Study the drawing (mm; zero at the part's minimum x, y, z) and answer. A direction names the side the tool comes from. Round coordinates to 2 decimals unless told otherwise and drop trailing zeros. Write each loop counter-clockwise with the first axis right and the second up, starting at its lowest first coordinate (ties: lowest second). Pieces come first, ordered by that corner, then holes. Notation, with made-up numbers: (-17, -35.75) - (-13, -35.75) arc R23 ccw to (-13, -6.75) - close; hole circle Ø10 at (53, 8). An arc over 180 degrees is marked (long way). Use one line per item in the form item = value. Start each with the question number.
1) The part is cut by section B-B, the plane y = 18. Give the vertices of the cut face in (x, z), plus the area to 3 significant figures.
2) This flat-tipped pin is pushed along its axis until it touches: pin 1 (11 mm diameter, centred on x = 30, z = 7.5, fed in from +Y). Where does it stop, or does it pass through?
3) The part is cut by section D-D, the plane x = 112.5. Give the vertices of the cut face in (y, z).
4) Consider line 1 along X through (y, z) = (85.5, 46); line 2 along X through (y, z) = (32.5, 38); line 3 along X through (y, z) = (59, 7.5). Determine where each line is inside the solid, lowest interval first. Write a range as from..to.
5) The part is cut by section A-A, the plane x = 43. Give the vertices of the cut face in (y, z), plus the area to 3 significant figures.
6) For the marked faces 4, 5 and 6, determine the directions among +Z, -Z, +X, -X, +Y, -Y from which every point of the face is accessible in a straight line to the end or side of a thin tool.
7) The part is cut by section C-C, the plane z = 35. Give the vertices of the cut face in (x, y).
8) For a pull along Z with two mould halves and no side action, classify the marked faces 1, 2 and 3 as released by +Z, released by -Z, zero draft, split by the parting line, or undercut.
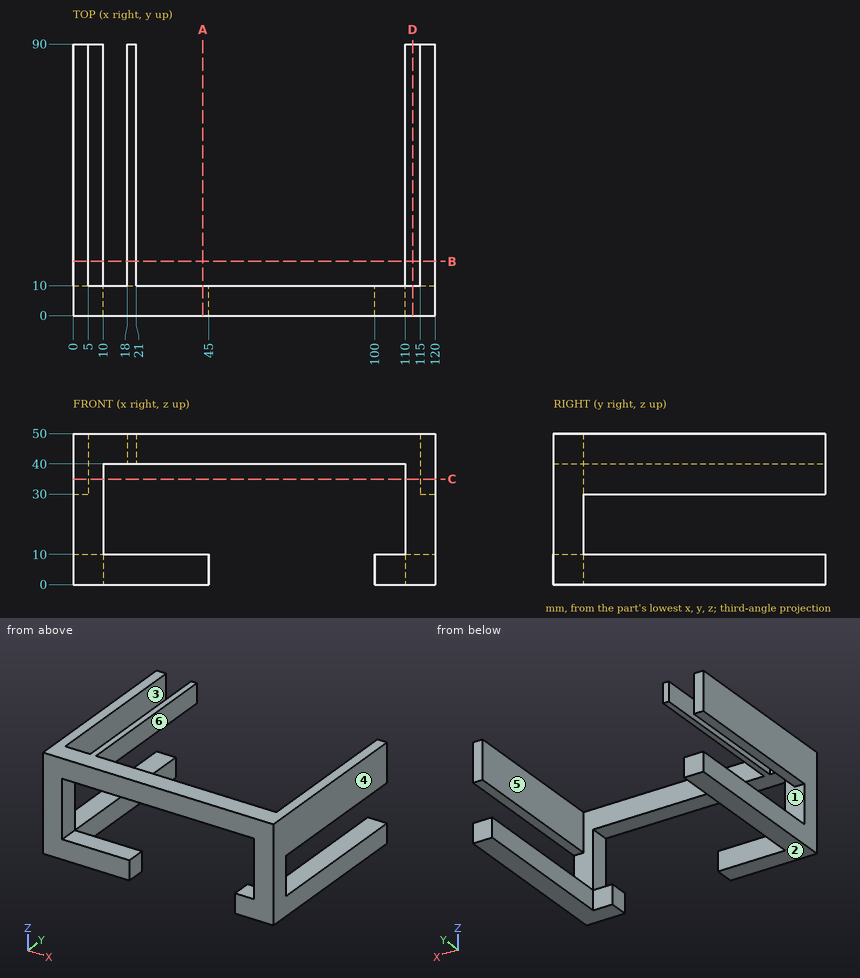
Geometry results:
q1.outline = (0, 0) - (10, 0) - (10, 10) - (0, 10) - close; (0, 30) - (5, 30) - (5, 50) - (0, 50) - close; (18, 40) - (21, 40) - (21, 50) - (18, 50) - close; (110, 0) - (120, 0) - (120, 10) - (110, 10) - close; (115, 30) - (120, 30) - (120, 50) - (115, 50) - close
q1.area = 430 mm2
q2.pin_1 = 10
q3.outline = (0, 0) - (90, 0) - (90, 10) - (10, 10) - (10, 50) - (0, 50) - close
q4.line_1 = 0..5, 18..21, 115..120
q4.line_2 = 0..5, 115..120
q4.line_3 = 0..10, 110..120
q5.outline = (0, 0) - (10, 0) - (10, 10) - (0, 10) - close; (0, 40) - (10, 40) - (10, 50) - (0, 50) - close
q5.area = 200 mm2
q6.face_4 = +Z, -Z, +X, +Y, -Y
q6.face_5 = +Z, +Y
q6.face_6 = +Z, -Z, +Y
q7.outline = (0, 0) - (10, 0) - (10, 10) - (5, 10) - (5, 90) - (0, 90) - close; (110, 0) - (120, 0) - (120, 90) - (115, 90) - (115, 10) - (110, 10) - close
q8.face_1 = undercut
q8.face_2 = released by -Z
q8.face_3 = zero draft
